Design review of the part built by this model. Coordinates are the model's own, in mm. Face numbers are marked on the shaded views. Give positions to 0.01 mm unless a question says otherwise; leave off trailing zeros. Loops run counter-clockwise (first coordinate to the right, second up) from the corner with the lowest first, then second, coordinate; pieces in that order, holes last. Notation, with made-up numbers: (3, 23.25) - (39, 23.25) arc R31 ccw to (39, 49.25) - close; hole circle Ø5 at (2, -32). An arc over 180 degrees is marked (long way). One line per item, written item: value. Start each with the question number.
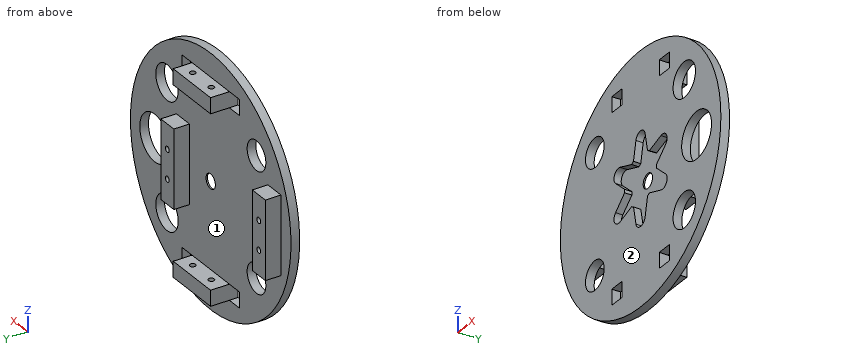
```python
from build123d import *

# Parameters (mm, degrees)
CROQUIS1_R              = 42.989543869
CROQUIS1_R_2            = 8.000000719
CROQUIS1_R_3            = 6.000000354
CROQUIS1_R_4            = 4.999998849
CROQUIS1_R_5            = 5.000081965
CROQUIS1_R_6            = 6.000000031
CROQUIS1_W              = 5.400000572
CROQUIS1_H              = 5.400000573
CROQUIS1_W_2            = 5.400001526
CROQUIS1_H_2            = 5.400001526
CROQUIS1_W_3            = 5.400001525
SALIENTE_EXTRUIR1_DEPTH = 2.5
CROQUIS2_R              = 42.989543869
CROQUIS2_R_2            = 5.000081965
CROQUIS2_R_3            = 6.000000031
CROQUIS2_R_4            = 8.000000719
CROQUIS2_R_5            = 6.000000354
CROQUIS2_R_6            = 4.999998849
CROQUIS2_R_7            = 2.5
CROQUIS2_W              = 5.400000572
CROQUIS2_H              = 5.400000573
CROQUIS2_W_2            = 5.400001525
CROQUIS2_H_2            = 5.400001526
CROQUIS2_W_3            = 5.400001526
SALIENTE_EXTRUIR2_DEPTH = 0.5
CROQUIS3_W              = 19.999999047
CROQUIS3_H              = 5.400000573
CROQUIS3_W_2            = 19.999998093
CROQUIS3_H_2            = 5.400001526
SALIENTE_EXTRUIR3_DEPTH = 6.5
CROQUIS4_R              = 1
CORTAR_EXTRUIR1_DEPTH   = 94.5
CROQUIS5_W              = 7.000000953
CROQUIS5_H              = 27
CROQUIS5_R              = 1.000001566
CROQUIS5_W_2            = 7.000000954
SALIENTE_EXTRUIR4_DEPTH = 5.4


with BuildPart() as part:
    # Croquis1 → Saliente-Extruir1 (new body)
    with BuildSketch(Plane(origin=(0, 0, 0), x_dir=(1, 0, 0), z_dir=(0, 1, 0))):
        with Locations((0.133743246, 0.231297164)):
            Circle(CROQUIS1_R)
        with Locations((30.123277351, 0.24111594)):
            Circle(CROQUIS1_R_2, mode=Mode.SUBTRACT)
        with Locations((23.52660556, 22.065066477)):
            Circle(CROQUIS1_R_3, mode=Mode.SUBTRACT)
        with Locations((-24.390140184, 20.810319956)):
            Circle(CROQUIS1_R_4, mode=Mode.SUBTRACT)
        with Locations((-24.392687184, -20.328024023)):
            Circle(CROQUIS1_R_5, mode=Mode.SUBTRACT)
        with Locations((23.526602762, -21.582829156)):
            Circle(CROQUIS1_R_6, mode=Mode.SUBTRACT)
        with BuildLine():
            Line((4.854387983, 7.302748706), (11.022837385, 9.362418202))
            ThreePointArc((11.022837385, 9.362418202), (13.987829641, 8.239301442), (13.466977705, 5.11179707))
            Line((13.466977705, 5.11179707), (8.599027265, 0.799598431))
            ThreePointArc((8.599027265, 0.799598431), (8.617971382, 0.221716337), (8.597699336, -0.356120697))
            Line((8.597699336, -0.356120697), (13.465650144, -4.668319833))
            ThreePointArc((13.465650144, -4.668319833), (13.975498626, -7.797636828), (11.006574422, -8.910318006))
            Line((11.006574422, -8.910318006), (4.838125635, -6.850648581))
            ThreePointArc((4.838125635, -6.850648581), (4.347137119, -7.155995714), (3.836579545, -7.427358125))
            Line((3.836579545, -7.427358125), (2.536080952, -13.799226756))
            ThreePointArc((2.536080952, -13.799226756), (0.080937178, -15.805426992), (-2.36713509, -13.790603798))
            Line((-2.36713509, -13.790603798), (-3.667633438, -7.418735734))
            ThreePointArc((-3.667633438, -7.418735734), (-4.177566071, -7.146200773), (-4.667851599, -6.839726149))
            Line((-4.667851599, -6.839726149), (-10.836301, -8.899395645))
            ThreePointArc((-10.836301, -8.899395645), (-13.801293256, -7.776278885), (-13.28044132, -4.648774514))
            Line((-13.28044132, -4.648774514), (-8.41249088, -0.336575875))
            ThreePointArc((-8.41249088, -0.336575875), (-8.431434998, 0.24130622), (-8.411162951, 0.819143254))
            Line((-8.411162951, 0.819143254), (-13.279113759, 5.131342389))
            ThreePointArc((-13.279113759, 5.131342389), (-13.788962242, 8.260659385), (-10.820038037, 9.373340563))
            Line((-10.820038037, 9.373340563), (-4.65158925, 7.313671137))
            ThreePointArc((-4.65158925, 7.313671137), (-4.160600735, 7.619018271), (-3.65004316, 7.890380681))
            Line((-3.65004316, 7.890380681), (-2.349544567, 14.262249313))
            ThreePointArc((-2.349544567, 14.262249313), (0.105599207, 16.268449549), (2.553671475, 14.253626355))
            Line((2.553671475, 14.253626355), (3.854169823, 7.88175829))
            ThreePointArc((3.854169823, 7.88175829), (4.364102455, 7.60922333), (4.854387983, 7.302748706))
        make_face(mode=Mode.SUBTRACT)
        with Locations((-12.576717154, -32.008881065)):
            Rectangle(CROQUIS1_W, CROQUIS1_H, mode=Mode.SUBTRACT)
        with Locations((12.823282465, -32.008881065)):
            Rectangle(CROQUIS1_W, CROQUIS1_H, mode=Mode.SUBTRACT)
        with Locations((-12.576716677, 32.491118458)):
            Rectangle(CROQUIS1_W_2, CROQUIS1_H_2, mode=Mode.SUBTRACT)
        with Locations((12.823282942, 32.491118458)):
            Rectangle(CROQUIS1_W_3, CROQUIS1_H_2, mode=Mode.SUBTRACT)
    extrude(amount=SALIENTE_EXTRUIR1_DEPTH)

    # Croquis2 → Saliente-Extruir2 (add)
    with BuildSketch(Plane(origin=(0, 2.5, 0), x_dir=(1, 0, 0), z_dir=(0, 1, 0))):
        with Locations((0.133743246, 0.231297164)):
            Circle(CROQUIS2_R)
        with Locations((-24.392687184, -20.328024023)):
            Circle(CROQUIS2_R_2, mode=Mode.SUBTRACT)
        with Locations((23.526602762, -21.582829156)):
            Circle(CROQUIS2_R_3, mode=Mode.SUBTRACT)
        with Locations((30.123277351, 0.24111594)):
            Circle(CROQUIS2_R_4, mode=Mode.SUBTRACT)
        with Locations((23.52660556, 22.065066477)):
            Circle(CROQUIS2_R_5, mode=Mode.SUBTRACT)
        with Locations((-24.390140184, 20.810319956)):
            Circle(CROQUIS2_R_6, mode=Mode.SUBTRACT)
        with Locations((0.133743246, 0.231297164)):
            Circle(CROQUIS2_R_7, mode=Mode.SUBTRACT)
        with Locations((-12.576717154, -32.008881065)):
            Rectangle(CROQUIS2_W, CROQUIS2_H, mode=Mode.SUBTRACT)
        with Locations((12.823282465, -32.008881065)):
            Rectangle(CROQUIS2_W, CROQUIS2_H, mode=Mode.SUBTRACT)
        with Locations((12.823282942, 32.491118458)):
            Rectangle(CROQUIS2_W_2, CROQUIS2_H_2, mode=Mode.SUBTRACT)
        with Locations((-12.576716677, 32.491118458)):
            Rectangle(CROQUIS2_W_3, CROQUIS2_H_2, mode=Mode.SUBTRACT)
    extrude(amount=SALIENTE_EXTRUIR2_DEPTH)

    # Croquis3 → Saliente-Extruir3 (add)
    with BuildSketch(Plane(origin=(0, 3, 0), x_dir=(1, 0, 0), z_dir=(0, 1, 0))):
        with Locations((0.123282655, -32.008881065)):
            Rectangle(CROQUIS3_W, CROQUIS3_H)
        with Locations((0.123283133, 32.491118458)):
            Rectangle(CROQUIS3_W_2, CROQUIS3_H_2)
    extrude(amount=SALIENTE_EXTRUIR3_DEPTH)

    # Croquis4 → Cortar-Extruir1 (cut)
    with BuildSketch(Plane.XY.offset(34.708881352)):
        with Locations((-4.876716868, 6)):
            Circle(CROQUIS4_R)
        with Locations((5.123283132, 6)):
            Circle(CROQUIS4_R)
    extrude(amount=-CORTAR_EXTRUIR1_DEPTH, mode=Mode.SUBTRACT)

    # Croquis5 → Saliente-Extruir4 (add)
    with BuildSketch(Plane(origin=(0, 3, 0), x_dir=(1, 0, 0), z_dir=(0, 1, 0))):
        with Locations((-34.010001431, 0)):
            Rectangle(CROQUIS5_W, CROQUIS5_H)
        with Locations((-34.010010931, 4.999991869)):
            Circle(CROQUIS5_R, mode=Mode.SUBTRACT)
        with Locations((-34.010010931, -4.999998876)):
            Circle(CROQUIS5_R, mode=Mode.SUBTRACT)
        with Locations((14.990000477, 0)):
            Rectangle(CROQUIS5_W_2, CROQUIS5_H)
        with Locations((14.989999497, 4.999991869)):
            Circle(CROQUIS5_R, mode=Mode.SUBTRACT)
        with Locations((14.989999497, -4.999998876)):
            Circle(CROQUIS5_R, mode=Mode.SUBTRACT)
    extrude(amount=SALIENTE_EXTRUIR4_DEPTH)


solid = part.part
```
(1) For pin 1 Ø2.5 at (y, z) = (5.5, 3.5) entering from -X; pin 2 Ø2.5 at (x, y) = (-4.88, 6) entering from +Z; pin 3 Ø3 at (x, z) = (-4, 4) entering from +Y, all flat-tipped, find the tip position at first contact; note any pin that passes through.
(2) To check wall thickness, follow L1, parallel to X at y = 1.25, z = -34.5; L2, parallel to Z at x = -9.5, y = 9; L3, parallel to X at y = 8, z = 11.5. State the ranges of each line that lie inside material, in increasing order. Write a range as from..to.
(3) Take a section at B-B on y = 6. State how many separate pieces and enclosed holes the cut face has, and give its area (3 significant figures).
(4) Take a section at C-C on z = 36. State the section outline as (x, y) points.
(5) Draft analysis for pull direction Z (two halves, no side actions). For the marked faces 1 and 2, state which applies: pulls with the +Z half, pulls with the -Z half, needs draft (parallel to the pull), parting line crosses it, or undercut.
(6) Take a section at A-A on x = -22. State the section outline as (y, z) points, and give its area (3 significant figures).
Here are the results:
1. pin 1: x = -37.51
1. pin 2: z = 34.71
1. pin 3: y = 3
2. L1: -25.82..-15.28, -9.88..10.12, 15.52..26.09
2. L2: -35.19..-29.79, 29.31..34.71
2. L3: -37.51..-30.51, 11.49..18.49
3. separate pieces: 8
3. enclosed holes: 4
3. area: 538 mm²
4. outline: (-23, 0) - (23.27, 0) - (23.27, 3) - (-23, 3) - close
5. face 1: undercut
5. face 2: needs draft
6. outline: (0, -37.09) - (3, -37.09) - (3, -25.2) - (0, -25.2) - close; (0, -16.42) - (3, -16.42) - (3, 15.94) - (0, 15.94) - close; (0, 24.72) - (3, 24.72) - (3, 36.62) - (0, 36.62) - close
6. area: 168 mm²
